The listing builds one solid part. Answer for the finished solid, in the listing's coordinates (mm). Face numbers are marked on the shaded views. Round coordinates to 2 decimals unless told otherwise and drop trailing zeros. Write each loop counter-clockwise with the first axis right and the second up, starting at its lowest first coordinate (ties: lowest second). Pieces come first, ordered by that corner, then holes. Notation, with made-up numbers: (80.5, -8.75) - (129.5, -8.75) arc R12 cw to (129.5, 7.25) - close; hole circle Ø3 at (67, 7.25). An arc over 180 degrees is marked (long way). Use a Markdown table: item, result. Add a question column.
1) Find the intervals of material crossed by probe 1 along Y at (x, z) = (-2.61, 0.55); probe 2 along X at (y, z) = (-6.59, 0.5); probe 3 along Y at (x, z) = (5.5, 1.35), in increasing order. Write a range as from..to.
2) Determine the mould class of the marked faces 1, 2 and 3 for opening direction Y: +Y half, -Y half, draft (parallel to the pull), parting line (faces both ways), or undercut.
3) This flat-tipped pin is pushed along its axis until it touches: P1, Ø3.5, axis at x = 6.35, y = 6.35, coming from the +Z side. Where does it stop, or does it pass through?
4) A cutting plane is placed at B-B (z = 1.35). Give the vertices of the cut face in (x, y), then the cut area to 3 significant figures.
5) A cutting plane is placed at D-D (y = -6.59). Give the vertices of the cut face in (x, z), then the cut area to 3 significant figures.
6) A cutting plane is placed at C-C (y = 6.75). Give the vertices of the cut face in (x, z), then the cut area to 3 significant figures.
7) A cutting plane is placed at A-A (x = -0.03). Give the vertices of the cut face in (y, z).
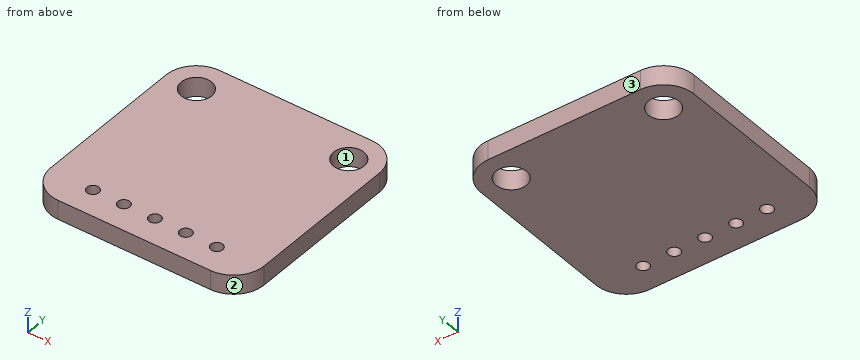
```python
from build123d import *

# Parameters (mm, degrees)
SKETCH2_R               = 1.27
BOSS_EXTRUDE1_DEPTH     = 1.6
CUT_EXTRUDE1_DEPTH      = 13.673760294
CUT_EXTRUDE1_DEPTH_BACK = 13.673760294
SKETCH3_R               = 0.5


with BuildPart() as part:
    # Sketch2 → Boss-Extrude1 (new body)
    with BuildSketch(Plane.XY):
        with BuildLine():
            Line((-6.35, -8.89), (6.35, -8.89))
            ThreePointArc((6.35, -8.89), (8.146051224, -8.146051224), (8.89, -6.35))
            Line((8.89, -6.35), (8.89, 6.35))
            ThreePointArc((8.89, 6.35), (8.146051224, 8.146051224), (6.35, 8.89))
            Line((6.35, 8.89), (-6.35, 8.89))
            ThreePointArc((-6.35, 8.89), (-8.146051224, 8.146051224), (-8.89, 6.35))
            Line((-8.89, 6.35), (-8.89, -6.35))
            ThreePointArc((-8.89, -6.35), (-8.146051224, -8.146051224), (-6.35, -8.89))
        make_face()
        with Locations((-6.35, 6.35)):
            Circle(SKETCH2_R, mode=Mode.SUBTRACT)
        with Locations((6.35, 6.35)):
            Circle(SKETCH2_R, mode=Mode.SUBTRACT)
    extrude(amount=BOSS_EXTRUDE1_DEPTH)

    # Sketch3 → Cut-Extrude1 (cut, two sides: drawn at the far end of the back side and taken through both)
    with BuildSketch(Plane.XY.offset(1.6).offset(-CUT_EXTRUDE1_DEPTH_BACK)):
        with Locations((-5.19, -6.59)):
            Circle(SKETCH3_R)
        with Locations((-2.61, -6.59)):
            Circle(SKETCH3_R)
        with Locations((-0.03, -6.59)):
            Circle(SKETCH3_R)
        with Locations((2.55, -6.59)):
            Circle(SKETCH3_R)
        with Locations((5.13, -6.59)):
            Circle(SKETCH3_R)
    extrude(amount=CUT_EXTRUDE1_DEPTH + CUT_EXTRUDE1_DEPTH_BACK, mode=Mode.SUBTRACT)


solid = part.part
```
Entries:
| question | item | result |
|---|---|---|
| 1 | probe 1 | y = -8.89..-7.09, -6.09..8.89 |
| 1 | probe 2 | x = -8.88..-5.69, -4.69..-3.11, -2.11..-0.53, 0.47..2.05, 3.05..4.63, 5.63..8.88 |
| 1 | probe 3 | y = -8.89..-6.93, -6.25..5.41, 7.29..8.89 |
| 2 | face 1 | undercut |
| 2 | face 2 | -Y half |
| 2 | face 3 | +Y half |
| 3 | P1 | stops at z = 1.6 |
| 4 | outline | (-8.89, -6.35) arc R2.54 ccw to (-6.35, -8.89) - (6.35, -8.89) arc R2.54 ccw to (8.89, -6.35) - (8.89, 6.35) arc R2.54 ccw to (6.35, 8.89) - (-6.35, 8.89) arc R2.54 ccw to (-8.89, 6.35) - close; hole circle Ø2.54 at (-6.35, 6.35); hole circle Ø1 at (-5.19, -6.59); hole circle Ø1 at (-2.61, -6.59); hole circle Ø1 at (-0.03, -6.59); hole circle Ø1 at (2.55, -6.59); hole circle Ø1 at (5.13, -6.59); hole circle Ø2.54 at (6.35, 6.35) |
| 4 | area | 297 mm² |
| 5 | outline | (-8.88, 0) - (-5.69, 0) - (-5.69, 1.6) - (-8.88, 1.6) - close; (-4.69, 0) - (-3.11, 0) - (-3.11, 1.6) - (-4.69, 1.6) - close; (-2.11, 0) - (-0.53, 0) - (-0.53, 1.6) - (-2.11, 1.6) - close; (0.47, 0) - (2.05, 0) - (2.05, 1.6) - (0.47, 1.6) - close; (3.05, 0) - (4.63, 0) - (4.63, 1.6) - (3.05, 1.6) - close; (5.63, 0) - (8.88, 0) - (8.88, 1.6) - (5.63, 1.6) - close |
| 5 | area | 20.4 mm² |
| 6 | outline | (-8.86, 0) - (-7.56, 0) - (-7.56, 1.6) - (-8.86, 1.6) - close; (-5.14, 0) - (5.14, 0) - (5.14, 1.6) - (-5.14, 1.6) - close; (7.56, 0) - (8.86, 0) - (8.86, 1.6) - (7.56, 1.6) - close |
| 6 | area | 20.6 mm² |
| 7 | outline | (-8.89, 0) - (-7.09, 0) - (-7.09, 1.6) - (-8.89, 1.6) - close; (-6.09, 0) - (8.89, 0) - (8.89, 1.6) - (-6.09, 1.6) - close |
